```python
from build123d import *

# Parameters (mm, degrees)
CROQUIS1_R              = 18
SALIENTE_EXTRUIR1_DEPTH = 3
CROQUIS2_R              = 5.45
SALIENTE_EXTRUIR2_DEPTH = 2.6
CHAFL_N1_SIZE           = 0.5
REDONDEO1_R             = 0.5
CORTAR_EXTRUIR1_DEPTH   = 3
MATRIZC1_COUNT          = 8
CROQUIS4_R              = 4.05
CORTAR_EXTRUIR2_DEPTH   = 27.064535292


with BuildPart() as part:
    # Croquis1 → Saliente-Extruir1 (new body)
    with BuildSketch(Plane(origin=(0, 0, 0), x_dir=(0, 1, 0), z_dir=(0, 0, 1))):
        with Locations(Location((0, 0, 0), (0, 0, 270))):
            Circle(CROQUIS1_R)
    extrude(amount=SALIENTE_EXTRUIR1_DEPTH)

    # Croquis2 → Saliente-Extruir2 (add)
    with BuildSketch(Plane.XY.offset(3)):
        Circle(CROQUIS2_R)
    extrude(amount=SALIENTE_EXTRUIR2_DEPTH)

    # Chaflán1
    chafl_n1_edges = [part.edges().sort_by_distance(p)[0] for p in [
        (-18, 0, 3),
        (-5.45, 0, 5.6),
    ]]
    chamfer(chafl_n1_edges, length=CHAFL_N1_SIZE)

    # Redondeo1
    redondeo1_edges = [part.edges().sort_by_distance(p)[0] for p in [
        (-5.45, 0, 3),
    ]]
    fillet(redondeo1_edges, radius=REDONDEO1_R)

    # Croquis3 → Cortar-Extruir1 (cut)
    with BuildSketch(Plane.XY.offset(3)):
        Polygon((-4.041451884, 11.5), (-2.020725942, 8), (2.020725942, 8), (4.041451884, 11.5), (2.020725942, 15), (-2.020725942, 15), align=None)
    cortar_extruir1 = extrude(amount=-CORTAR_EXTRUIR1_DEPTH, mode=Mode.SUBTRACT)

    # MatrizC1: Cortar-Extruir1 ×8 about axis
    matrizc1_axis = Axis((0, 0, 0), (0, 0, 1))
    for i in range(1, MATRIZC1_COUNT):
        add(cortar_extruir1.rotate(matrizc1_axis, i * 360 / MATRIZC1_COUNT), mode=Mode.SUBTRACT)

    # Croquis4 → Cortar-Extruir2 (cut, through all)
    with BuildSketch(Plane.XY.offset(5.6)):
        Circle(CROQUIS4_R)
    extrude(amount=-CORTAR_EXTRUIR2_DEPTH, mode=Mode.SUBTRACT)


solid = part.part
```
Input: part model. Units: mm. Frame: model coordinates. Coordinates: 2 decimals unless noted, no trailing zeros. Order: outer loops, then holes, each group sorted by start corner. A loop starts at its lowest first (then second) coordinate and runs counter-clockwise, first axis right, second up. Notation, with made-up numbers: (58, 19) - (86, 19) arc R20 ccw to (86, 47) - close; hole circle Ø11 at (-13.75, 78). An arc over 180 degrees is marked (long way). Put each result on its own line as item: value.
1. Contact query for flat-ended pins moving along their axis: pin 1 Ø1.5 at (x, z) = (4, 1) entering from -Y; pin 2 Ø1.5 at (x, z) = (-0.5, 2) entering from -Y; pin 3 Ø2.5 at (x, z) = (-1, 1) entering from +Y. Output: stop coordinate, or through.
Report:
pin 1: stops at y = -17.7
pin 2: stops at y = -18
pin 3: stops at y = 18
2. Cut plane C-C on z = 1.55. State how many separate pieces and enclosed holes the cut face has, then the cut area to 3 significant figures.
Report:
separate pieces: 1
enclosed holes: 9
area: 627 mm2
3. Line query: line 1 along Y through (x, z) = (0, 1.55); line 2 along X through (y, z) = (-1.5, 2.25); line 3 along Y through (x, z) = (-5.5, 1.3). Output: solid intervals per line, ascending.
Report:
line 1: y = -18 to -15, -8 to -4.05, 4.05 to 8, 15 to 18
line 2: x = -17.94 to -15, -8 to -3.76, 3.76 to 8, 15 to 17.94
line 3: y = -17.14 to -11.05, -5.81 to 5.81, 11.05 to 17.14
4. Draft query along X for faces 1 (the face through (7.5, 0.2, 3)), 2 (the face through (9.01, 4.744, 1.521)). Return one class per face: pulls with the +X half, pulls with the -X half, needs draft (parallel to the pull), parting line crosses it, or undercut.
Report:
face 1: needs draft
face 2: undercut
5. Cut plane A-A on x = 0. Return the cut outline in (y, z).
Report:
outline: (-18, 0) - (-15, 0) - (-15, 3) - (-17.5, 3) - (-18, 2.5) - close; (-8, 0) - (-4.05, 0) - (-4.05, 5.6) - (-4.95, 5.6) - (-5.45, 5.1) - (-5.45, 3.5) arc R0.5 cw to (-5.95, 3) - (-8, 3) - close; (4.05, 0) - (8, 0) - (8, 3) - (5.95, 3) arc R0.5 cw to (5.45, 3.5) - (5.45, 5.1) - (4.95, 5.6) - (4.05, 5.6) - close; (15, 0) - (18, 0) - (18, 2.5) - (17.5, 3) - (15, 3) - close
